The listing builds one solid part. Answer for the finished solid, in the listing's coordinates (mm). A direction names the side the tool comes from. Round coordinates to 2 decimals unless told otherwise and drop trailing zeros. Write each loop counter-clockwise with the first axis right and the second up, starting at its lowest first coordinate (ties: lowest second). Pieces come first, ordered by that corner, then holes. Notation, with made-up numbers: M 46.5,-30.5 L 68.5,-30.5 A32 ccw 68.5,5.5 Z; hole C 24,59 d1. An arc over 180 degrees is marked long. Put each result on its own line as item: value. Start each with the question number.
```python
from build123d import *

# Parameters (mm, degrees)
SKETCH_1_R          = 1.5
SKETCH_1_W          = 4
SKETCH_1_H          = 8
SKETCH_1_R_2        = 4.1
SKETCH_1_R_3        = 11.1
EXTRUDE_6_DEPTH     = 5
SKETCH_2_R          = 2
CUT_EXTRUDE_1_DEPTH = 10


with BuildPart() as part:
    # 草图1 → 凸台-拉伸6 (new body)
    with BuildSketch(Plane(origin=(0, 0, 0), x_dir=(1, 0, 0), z_dir=(0, 1, 0))):
        Polygon((75, 150), (37.5, 150), (0, 150), (0, 0), (75, 0), align=None)
        with Locations((6, 10.5)):
            Circle(SKETCH_1_R, mode=Mode.SUBTRACT)
        with Locations((12.5, 10.5)):
            Rectangle(SKETCH_1_W, SKETCH_1_H, mode=Mode.SUBTRACT)
        with Locations((18.5, 10.5)):
            Circle(SKETCH_1_R, mode=Mode.SUBTRACT)
        with Locations((30.5, 10.5)):
            Circle(SKETCH_1_R, mode=Mode.SUBTRACT)
        with Locations((44.5, 10.5)):
            Circle(SKETCH_1_R, mode=Mode.SUBTRACT)
        with Locations((56.5, 10.5)):
            Circle(SKETCH_1_R, mode=Mode.SUBTRACT)
        with Locations((62.5, 10.5)):
            Rectangle(SKETCH_1_W, SKETCH_1_H, mode=Mode.SUBTRACT)
        with Locations((69, 10.5)):
            Circle(SKETCH_1_R, mode=Mode.SUBTRACT)
        with Locations((37.5, 132.25)):
            Circle(SKETCH_1_R_2, mode=Mode.SUBTRACT)
        with Locations((37.5, 113)):
            Circle(SKETCH_1_R_3, mode=Mode.SUBTRACT)
    extrude(amount=EXTRUDE_6_DEPTH)

    # 草图2 → 切除-拉伸1 (cut)
    with BuildSketch(Plane(origin=(0, 5, 0), x_dir=(1, 0, 0), z_dir=(0, 1, 0))):
        with Locations((37.5, 142)):
            Circle(SKETCH_2_R)
        with Locations((62.61473671, 98.5)):
            Circle(SKETCH_2_R)
        with Locations((12.38526329, 98.5)):
            Circle(SKETCH_2_R)
    extrude(amount=-CUT_EXTRUDE_1_DEPTH, mode=Mode.SUBTRACT)


solid = part.part
```
Item 1: Which of the six approach directions +Z, -Z, +X, -X, +Y, -Y give full straight-line access (tool end or side, diameter ignored) to faces 1 (the flat face through (37, 0, -76)), 2 (the flat face through (12, 2, -6.5))?
Item 2: Section C-C (z = -132.25) is taken. Give the vertices of the cut face in (x, y), and give its area (3 significant figures).
Item 3: Section A-A (z = -98.5) is taken. Give the vertices of the cut face in (x, y), and give its area (3 significant figures).
Item 4: Flat-ended cylindrical pins translate along their axes: pin 1 (2.5 mm diameter, centred on x = 6, z = -10.5, fed in from -Y); pin 2 (1.2 mm diameter, centred on x = 62, y = 2, fed in from +Z). Find the tip coordinate at first contact, or state that the pin passes through.
Item 5: Section B-B (x = 37.5) is taken. Give the vertices of the cut face in (y, z).
Item 6: Determine the mould class of faces 3 (the flat face through (37, 5, -76)), 4 (the flat face through (0, 2, -76)), 5 (the flat face through (62, 2, -14.5)) for opening direction X: released by +X, released by -X, zero draft, split by the parting line, or undercut.
Item 7: Consider line 1 along Z through (x, y) = (37.5, 1.75); line 2 along Z through (x, y) = (56.5, 3.65); line 3 along Z through (x, y) = (63, 0.9). Determine where each line is inside the solid, lowest interval first. Write a range as [from, to].
Item 8: Section D-D (x = 6) is taken. Give the vertices of the cut face in (y, z).
Output values:
1. face 1: +Z, -Z, +X, -X, -Y
1. face 2: +Y, -Y
2. outline: M 0,0 L 33.4,0 L 33.4,5 L 0,5 Z; M 41.6,0 L 75,0 L 75,5 L 41.6,5 Z
2. area: 334 mm^2
3. outline: M 0,0 L 10.39,0 L 10.39,5 L 0,5 Z; M 14.39,0 L 60.61,0 L 60.61,5 L 14.39,5 Z; M 64.61,0 L 75,0 L 75,5 L 64.61,5 Z
3. area: 335 mm^2
4. pin 1: passes through
4. pin 2: stops at z = 0
5. outline: M 0,-150 L 5,-150 L 5,-144 L 0,-144 Z; M 0,-140 L 5,-140 L 5,-136.35 L 0,-136.35 Z; M 0,-128.15 L 5,-128.15 L 5,-124.1 L 0,-124.1 Z; M 0,-101.9 L 5,-101.9 L 5,0 L 0,0 Z
6. face 3: zero draft
6. face 4: released by -X
6. face 5: undercut
7. line 1: z = [-150, -144], [-140, -136.35], [-128.15, -124.1], [-101.9, 0]
7. line 2: z = [-150, -12], [-9, 0]
7. line 3: z = [-150, -100.46], [-96.54, -14.5], [-6.5, 0]
8. outline: M 0,-150 L 5,-150 L 5,-12 L 0,-12 Z; M 0,-9 L 5,-9 L 5,0 L 0,0 Z
